Solid Edge part; units mm, degrees
sketch "Sketch1" plane through (0, 0, 0) normal (0, 0, 1) x (1, 0, 0)
  line L0 (0, 0) -> (-100, 0)
  line L1 (-100, 0) -> (-100, -35.4)
  line L2 (-100, -35.4) -> (0, -35.4)
  line L3 (0, -35.4) -> (0, 0)
extrude "Protrusion1" add sketch "Sketch1" against normal blind 30
sketch "Sketch2" plane through (-50, -17.7, 0) normal (0, 0, 1) x (1, 0, 0)
  line L0 (3, 7.7) -> (3, -7.3)
  arc A0 (-7, -7.3) -> (3, -7.3) centre (-2, -7.3) ccw
  line L1 (-7, -7.3) -> (-7, 7.7)
  arc A1 (-7, 7.7) -> (3, 7.7) centre (-2, 7.7) cw
extrude "ExtrudedCutout_1" cut sketch "Sketch2" against normal blind 30
fillet "Round_1" radius 30 1 edges at (0, -35.4, -15)
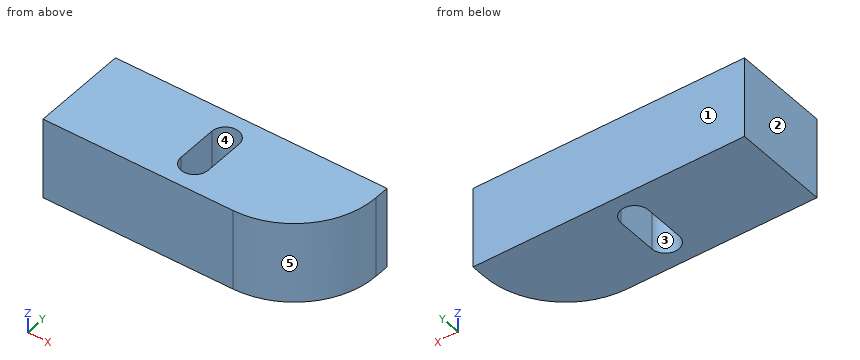
Check sheet for the modelled part. Datum: model origin and axes. Units: mm. Face numbers are marked on the shaded views. A direction names the side the tool comes from. Round coordinates to 2 decimals unless told otherwise and drop trailing zeros. Loops run counter-clockwise (first coordinate to the right, second up) from the corner with the lowest first, then second, coordinate; pieces in that order, holes last. Notation, with made-up numbers: (-5.75, 47.25) - (43.25, 47.25) arc R27 cw to (43.25, 68.25) - close; hole circle Ø6 at (-16.5, 46.5). An arc over 180 degrees is marked (long way). Answer as CSV lines item,"result". Start each with the question number.
Item 1: Release check for a two-part mould opening along Y. For the marked faces 1, 2 and 3 record: +Y half, -Y half, draft (parallel to the pull), parting line (faces both ways), or undercut.
Item 2: Section check C-C (y = -9). Record the boundary of the cut face in (x, z), and give its area (3 significant figures).
Item 3: Set-up check for the marked faces 4 and 5: record each of +Z, -Z, +X, -X, +Y, -Y from which the full face is reachable in a straight line by a thin tool's end or side.
Item 4: Depth check by flat-ended pin: P1, Ø2, axis at x = -45, y = -4.5, coming from the +Z side; P2, Ø2, axis at y = -19.5, z = -17.5, coming from the +X side; P3, Ø10, axis at y = -28.5, z = -5, coming from the +X side; P4, Ø1.5, axis at y = -9.5, z = -7, coming from the +X side. Enter the tip coordinate at first touch or a pass-through.
Item 5: Section check D-D (x = -19.5). Record the boundary of the cut face in (y, z), and give its area (3 significant figures).
Item 6: Section check A-A (x = -52). Record the boundary of the cut face in (y, z).
Item 7: Section check B-B (z = -28). Record the boundary of the cut face in (x, y).
Item 8: Scan lines: line 1 (X direction, y = -25, z = -13.75); line 2 (X direction, y = -22.5, z = -26); line 3 (Y direction, x = -23.5, z = -22.5). Record each from-to range of solid material in increasing order. Write a range as [from, to].
Report:
1,face 1,"+Y half"
1,face 2,"draft"
1,face 3,"undercut"
2,outline,"(-100, -30) - (-56.9, -30) - (-56.9, 0) - (-100, 0) - close; (-47.1, -30) - (-0.22, -30) - (-0.22, 0) - (-47.1, 0) - close"
2,area,"2,700 mm2"
3,face 4,"+Z, -Z"
3,face 5,"+Z, -Z, +X, -Y"
4,P1,"stops at z = 0"
4,P2,"stops at x = -3.01"
4,P3,"stops at x = -6.08"
4,P4,"stops at x = -0.19"
5,outline,"(-33.5, -30) - (0, -30) - (0, 0) - (-33.5, 0) - close"
5,area,"1,010 mm2"
6,outline,"(-35.4, -30) - (-30, -30) - (-30, 0) - (-35.4, 0) - close; (-5, -30) - (0, -30) - (0, 0) - (-5, 0) - close"
7,outline,"(-100, -35.4) - (-30, -35.4) arc R30 ccw to (0, -5.4) - (0, 0) - (-100, 0) - close; hole (-57, -25) arc R5 ccw to (-47, -25) - (-47, -10) arc R5 ccw to (-57, -10) - close"
8,line 1,"x = [-100, -57], [-47, -7.29]"
8,line 2,"x = [-100, -57], [-47, -5.35]"
8,line 3,"y = [-34.69, 0]"
